Geometry: final body of the model. Coordinates: model frame, mm. Face numbers are marked on the shaded views. A direction names the side the tool comes from. Coordinates: 2 decimals unless noted, no trailing zeros. Order: outer loops, then holes, each group sorted by start corner. A loop starts at its lowest first (then second) coordinate and runs counter-clockwise, first axis right, second up. Notation, with made-up numbers: (70.5, -11.75) - (126.5, -11.75) arc R13 ccw to (126.5, 6.25) - close; hole circle Ø1 at (-2, 39). An arc over 180 degrees is marked (long way). Use a Markdown table: item, result. Add a question column.
```python
from build123d import *

# Parameters (mm, degrees)
F0_W     = 35
F0_H     = 15
F1_DEPTH = 14
F2_DEPTH = 24
F3_DEPTH = 30


with BuildPart() as f1:
    # F0 (on Top) → F1 (new body)
    with BuildSketch(Plane.XY):
        Polygon((0, 30), (0, 0), (15, 0), (15, 15), (15, 30), align=None)
        with Locations((32.5, 7.5)):
            Rectangle(F0_W, F0_H)
        with Locations((32.5, 22.5)):
            Rectangle(F0_W, F0_H)
    extrude(amount=F1_DEPTH)

    # F0 (on Top) → F2 (join)
    with BuildSketch(Plane.XY):
        with Locations((32.5, 22.5)):
            Rectangle(F0_W, F0_H)
    extrude(amount=F2_DEPTH)

    # F0 (on Top) → F3 (join)
    with BuildSketch(Plane.XY):
        Polygon((0, 30), (0, 0), (15, 0), (15, 15), (15, 30), align=None)
    extrude(amount=F3_DEPTH)


solid = f1.part
```
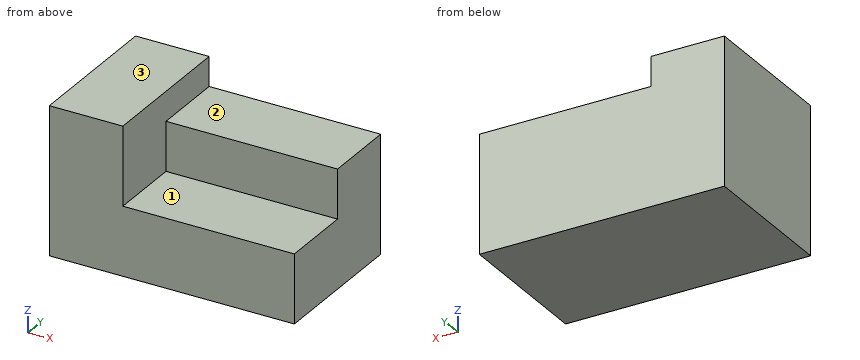
1) Section C-C (z = 26). Return loops of the section in (x, y).
2) Set-up query: the marked faces 1, 2 and 3. Return all of +Z, -Z, +X, -X, +Y, -Y with unobstructed straight access to the full face (end or side cutting, diameter ignored); none if empty.
3) Section B-B (x = 19). Return loops of the section in (y, z), then the cut area to 3 significant figures.
4) Ray query, line 1 along Y through (x, z) = (21.5, 15.75); line 2 along X through (y, z) = (6.5, 19.25); line 3 along Z through (x, y) = (39.5, 2.25). Return the intervals inside material, ascending.
5) Section A-A (z = 17). Return loops of the section in (x, y), then the cut area to 3 significant figures.
6) Pin query (flat end, axial travel): pin 1 (7.5 mm diameter, centred on x = 26, y = 7, fed in from +Z); pin 2 (4.5 mm diameter, centred on x = 41, y = 24, fed in from +Z); pin 3 (5 mm diameter, centred on x = 32, z = 18.5, fed in from -Y). Return the tip coordinate at first contact, or that it passes through.
Values follow:
| question | item | result |
|---|---|---|
| 1 | outline | (0, 0) - (15, 0) - (15, 30) - (0, 30) - close |
| 2 | face 1 | +Z, +X, -Y |
| 2 | face 2 | +Z, +X, +Y, -Y |
| 2 | face 3 | +Z, +X, -X, +Y, -Y |
| 3 | outline | (0, 0) - (30, 0) - (30, 24) - (15, 24) - (15, 14) - (0, 14) - close |
| 3 | area | 570 mm² |
| 4 | line 1 | y = 15 to 30 |
| 4 | line 2 | x = 0 to 15 |
| 4 | line 3 | z = 0 to 14 |
| 5 | outline | (0, 0) - (15, 0) - (15, 15) - (50, 15) - (50, 30) - (0, 30) - close |
| 5 | area | 975 mm² |
| 6 | pin 1 | stops at z = 14 |
| 6 | pin 2 | stops at z = 24 |
| 6 | pin 3 | stops at y = 15 |
